Model file for the job. Use its own axes, mm. A direction names the side the tool comes from. Give positions to 0.01 mm unless a question says otherwise; leave off trailing zeros. Loops run counter-clockwise (first coordinate to the right, second up) from the corner with the lowest first, then second, coordinate; pieces in that order, holes last. Notation, with made-up numbers: M 12.5,68.5 L 63.5,68.5 A28 cw 63.5,87.5 Z; hole C 4,-14.75 d6. An arc over 180 degrees is marked long. Answer in a Markdown table with one row per item.
```python
from build123d import *

# Parameters (mm, degrees)
F1_DEPTH = 25
F2_R     = 3
F3_DEPTH = 34.37407
F4_R     = 4.25
F5_DEPTH = 90.001


with BuildPart() as f1:
    # F0 (on Front) → F1 (new body)
    with BuildSketch(Plane.XZ):
        with BuildLine():
            Line((-25, 19.37307), (-45, 5))
            Line((-45, 5), (-45, 0))
            Line((-45, 0), (-45, -40))
            Line((-45, -40), (-35, -40))
            Line((-35, -40), (-30, -15))
            Line((-30, -15), (0, -15))
            Line((0, -15), (30, -15))
            Line((30, -15), (35, -40))
            Line((35, -40), (45, -40))
            Line((45, -40), (45, 0))
            Line((45, 0), (45, 5))
            Line((45, 5), (25, 19.37307))
            Line((25, 19.37307), (10, 19.37307))
            ThreePointArc((10, 19.37307), (0, 9.37307), (-10, 19.37307))
            Line((-10, 19.37307), (-25, 19.37307))
        make_face()
    extrude(amount=F1_DEPTH)

    # F2 (on face) → F3 (cut, through all)
    with BuildSketch(Plane(origin=(0, 0, -15), x_dir=(1, 0, 0), z_dir=(0, 0, -1))):
        with Locations((-16.9, 12.5)):
            Circle(F2_R)
        with Locations((16.9, 12.5)):
            Circle(F2_R)
    extrude(amount=-F3_DEPTH, mode=Mode.SUBTRACT)

    # F4 (on face) → F5 (cut, through all)
    with BuildSketch(Plane(origin=(-45, 0, 0), x_dir=(0, -1, 0), z_dir=(-1, 0, 0))):
        with Locations((12.5, -25.221726)):
            Circle(F4_R)
    extrude(amount=-F5_DEPTH, mode=Mode.SUBTRACT)


solid = f1.part
```
Q1. Saw through at B-B (z = -20). Give the cut face in (x, y).
Reported:
| item | result |
|---|---|
| outline | M -45,-25 L -31,-25 L -31,0 L -45,0 Z; M 31,-25 L 45,-25 L 45,0 L 31,0 Z |
Q2. Drop flat-ended pins along their axis: pin 1 (8 mm diameter, centred on x = -6, z = 9.5, fed in from +Y); pin 2 (3.5 mm diameter, centred on x = 16.9, y = -12.5, fed in from +Z); pin 3 (12 mm diameter, centred on x = -13, y = -19, fed in from -Z). Give the stop position or say it passes through.
Reported:
| item | result |
|---|---|
| pin 1 | y = 0 |
| pin 2 | through |
| pin 3 | z = -15 |
Q3. Saw through at A-A (x = 16.9). Give the cut face in (y, z).
Reported:
| item | result |
|---|---|
| outline | M -25,-15 L -15.5,-15 L -15.5,19.37 L -25,19.37 Z; M -9.5,-15 L 0,-15 L 0,19.37 L -9.5,19.37 Z |
Q4. Probe probe 1 along X at (y, z) = (-12.75, 5); probe 2 along Y at (x, z) = (-16.9, 0.5); probe 3 along X at (y, z) = (-12.5, 6). List the from-to ranges inside material, lowest first.
Reported:
| item | result |
|---|---|
| probe 1 | -45 to -19.89, -13.91 to 13.91, 19.89 to 45 |
| probe 2 | -25 to -15.5, -9.5 to 0 |
| probe 3 | -43.61 to -19.9, -13.9 to 13.9, 19.9 to 43.61 |
Q5. 3-axis set-ups, long thin cutter, end or side, ignore diameter. For faces 5 (the face through (0.22, -12.325, 9.375)), 6 (the face through (-33, -12, -30)): which of +Z, -Z, +X, -X, +Y, -Y reach the whole face in a straight line?
Reported:
| item | result |
|---|---|
| face 5 | +Z, +Y, -Y |
| face 6 | -Z, +Y, -Y |
Q6. Saw through at D-D (y = -6.25). Give the cut face in (x, z), and give its area (3 significant figures).
Reported:
| item | result |
|---|---|
| outline | M -45,-40 L -35,-40 L -30,-15 L 30,-15 L 35,-40 L 45,-40 L 45,5 L 25,19.37 L 10,19.37 A10 cw -10,19.37 L -25,19.37 L -45,5 Z |
| area | 3,270 mm² |
Q7. Mould opens along X. For faces 1 (the face through (-14.13, -11.35, 1.95)), 2 (the face through (-45, -12, -17)), 3 (the face through (-40, -12, -40)), 4 (the face through (35.14, -12.325, 12.086)) say: released by +X, released by -X, zero draft, split by the parting line, or undercut.
Reported:
| item | result |
|---|---|
| face 1 | undercut |
| face 2 | released by -X |
| face 3 | zero draft |
| face 4 | released by +X |
Q8. Saw through at C-C (y = -12.5). Give the cut face in (x, z), and give its area (3 significant figures).
Reported:
| item | result |
|---|---|
| outline | M -45,-40 L -35,-40 L -32.89,-29.47 L -45,-29.47 Z; M -45,-20.97 L -31.19,-20.97 L -30,-15 L -19.9,-15 L -19.9,19.37 L -25,19.37 L -45,5 Z; M -13.9,-15 L 13.9,-15 L 13.9,19.37 L 10,19.37 A10 cw -10,19.37 L -13.9,19.37 Z; M 19.9,-15 L 30,-15 L 31.19,-20.97 L 45,-20.97 L 45,5 L 25,19.37 L 19.9,19.37 Z; M 32.89,-29.47 L 35,-40 L 45,-40 L 45,-29.47 Z |
| area | 2,640 mm² |
